Model file for the job. Use its own axes, mm. A direction names the side the tool comes from. Coordinates: 2 decimals unless noted, no trailing zeros. Write each loop counter-clockwise with the first axis right and the second up, starting at its lowest first coordinate (ties: lowest second). Pieces come first, ordered by that corner, then holes. Notation, with made-up numbers: (34.25, 33) - (52.25, 33) arc R17 cw to (52.25, 57) - close; hole circle Ø7 at (36.5, -26). An arc over 180 degrees is marked (long way). Put each result on its own line as item: value. Start each with the question number.
1. Saw through at B-B, the plane y = -3. Write the cut outline in (x, z).
2. Saw through at C-C, the plane y = -12. Write the cut outline in (x, z), plus the area to 3 significant figures.
3. Drop flat-ended pins along their axis: P1, Ø2, axis at x = -13.5, z = 2.5, coming from the +Y side; P2, Ø2.5, axis at x = -63, z = 1.5, coming from the +Y side; P3, Ø3.5, axis at y = -1, z = 1, coming from the +X side. Give the stop position or say it passes through.
4. Which spindle directions (+Z, -Z, +X, -X, +Y, -Y) get a long thin tool onto all of the face, cutting with end or side? Do faces 1 (the face through (-47.167, -18.974, 4.972)), 2 (the face through (-5, 16, 1)), 3 (the face through (-75, -20, 1)). Say none if no direction does.
5. Drill centre lines: L1, parallel to Y at x = -93.5, z = 0.75; L2, parallel to Y at x = -109, z = 1; L3, parallel to X at y = -22, z = 1. Where is each one in solid material? Low to high. Write a range as from..to.
6. Saw through at A-A, the plane x = -36.5. Write the cut outline in (y, z), plus the area to 3 significant figures.
7. Pull direction X, two halves, no side cores. Call faces 4 (the face through (-106.49, 16.92, 4.97)), 5 (the face through (-45.997, -15.181, 1.479)), 6 (the face through (-120, 16, 1)), 7 (the face through (5.416, 12.94, 1.479)): released by +X, released by -X, zero draft, split by the parting line, or undercut.
Autodesk Inventor part; units mm, degrees
ref_plane "YZ Plane" through (0, 0, 0) normal (1, 0, 0) x (0, 1, 0)
ref_plane "XZ Plane" through (0, 0, 0) normal (0, 1, 0) x (-1, 0, 0)
ref_plane "XY Plane" through (0, 0, 0) normal (0, 0, 1) x (1, 0, 0)
sketch "Sketch1" plane through (0, 0, 0) normal (0, 0, 1) x (1, 0, 0)
  circle A0 centre (1.5276, -12) radius 1.75
  circle A1 centre (1.5276, 0) radius 1.75
  circle A2 centre (1.5276, 12) radius 1.75
  arc A3 (1.5276, -16) -> (3.2181, -8.3748) centre (1.5276, -12) ccw
  line L0 (3.2181, -8.3748) -> (-2.4724, -5.7213)
  line L1 (1.5276, -16) -> (-60.6, -16)
  line L2 (11.3984, 0) -> (-64.1078, 0)
  line L3 (-60.6, 141.7) -> (-60.6, -41.7)
  line L4 (-2.4724, -5.7213) -> (-2.4724, 0)
  arc A4 (3.2181, 8.3748) -> (1.5276, 16) centre (1.5276, 12) ccw
  line L5 (3.2181, 8.3748) -> (-2.4724, 5.7213)
  line L6 (1.5276, 16) -> (-60.6, 16) construction
  line L7 (-2.4724, 5.7213) -> (-2.4724, 0)
  circle A5 centre (-32.0875, 25.9484) radius 1.6
  circle A6 centre (-44.5875, -20.9516) radius 1.6
  circle A7 centre (-109.5875, -20.9516) radius 1.6
  circle A8 centre (-109.5875, 17.8984) radius 1.6
  line L8 (-30.6, -16) -> (-40.6, -26)
  line L9 (-30.6, -16) -> (-16.4579, -16) construction
  line L10 (-40.6, -26) -> (-60.6, -26)
  line L11 (1.5276, 16) -> (-23.224, 16)
  line L12 (-23.224, 16) -> (-31.224, 24) construction
  line L13 (-23.224, 16) -> (-11.9103, 16) construction
  line L14 (-31.224, 24) -> (-109.7276, 24)
  line L15 (-109.7276, 24) -> (-117.7276, 16)
  circle A9 centre (-122.7276, -12) radius 1.75
  circle A10 centre (-122.7276, 0) radius 1.75
  circle A11 centre (-122.7276, 12) radius 1.75
  arc A12 (-124.4181, -8.3748) -> (-122.7276, -16) centre (-122.7276, -12) ccw
  arc A13 (-122.7276, 16) -> (-124.4181, 8.3748) centre (-122.7276, 12) ccw
  line L16 (-122.7276, 16) -> (-117.7276, 16)
  line L17 (-60.6, -26) -> (-112.7276, -26)
  line L18 (-112.7276, -26) -> (-122.7276, -16)
  line L19 (-124.4181, -8.3748) -> (-118.7276, -5.7213)
  line L20 (-118.7276, -5.7213) -> (-118.7276, 0)
  line L21 (-118.7276, 5.7213) -> (-118.7276, 0)
  line L22 (-124.4181, 8.3748) -> (-118.7276, 5.7213)
  line L23 (-11.9103, 16) -> (-25.5298, 29.6196)
  line L24 (-11.9103, 16) -> (7.3507, 16) construction
  line L25 (-25.5298, 29.6196) -> (-40.2322, 29.6196)
  line L26 (-40.2322, 29.6196) -> (-45.8517, 24)
  line L27 (-12.954, -10.4954) -> (-41.3116, -10.4954)
  line L28 (-41.3116, -10.4954) -> (-50.8162, -20)
  line L29 (-50.8162, -20) -> (-99.9221, -20)
  line L30 (-99.9221, -20) -> (-110.7276, -9.1945)
  line L31 (-110.7276, -9.1945) -> (-110.7276, 3.4171)
  line L32 (-110.7276, 3.4171) -> (-98.1447, 16)
  line L33 (-98.1447, 16) -> (-21.5239, 16)
  line L34 (-21.5239, 16) -> (-17.2785, 11.7546)
  line L35 (-17.2785, 11.7546) -> (-17.448, 11.7546)
  line L36 (-17.448, 11.7546) -> (-8.8369, 3.1435)
  line L37 (-8.8369, 3.1435) -> (-8.8369, -6.3783)
  line L38 (-8.8369, -6.3783) -> (-12.954, -10.4954)
  point P0 (0, 0)
extrude "Extrusion1" add sketch "Sketch1" along normal blind 3 contours L4 L0 A3 L1 L28 L27 L38 L37 L2 | L2 L37 L36 L35 L34 L11 A4 L5 L7 | L33 L32 L31 L30 L29 L3 L17 L18 A12 L19 L20 L21 L22 A13 L16 L15 L14 | L3 L14 L26 L25 L23 L11 L33 | L1 L8 L10 L3 L29 L28
sketch "Sketch2" plane through (0, 0, 3) normal (0, 0, 1) x (1, 0, 0)
  circle A0 centre (-32.0875, 25.9484) radius 1.6
  circle A1 centre (-44.5875, -20.9516) radius 1.6
  circle A2 centre (-109.5875, -20.9516) radius 1.6
  circle A3 centre (-109.5875, 17.8984) radius 1.6
  circle A4 centre (-109.5875, -20.9516) radius 3.25
  circle A5 centre (-109.5875, 17.8984) radius 3.25
  circle A6 centre (-32.0875, 25.9484) radius 3.25
  circle A7 centre (-44.5875, -20.9516) radius 1.6
  circle A8 centre (-44.5875, -20.9516) radius 3.25
  point P0 (0, 0)
  dimension "d15" = 6.5
  dimension "d16" = 6.5
  dimension "d17" = 6.5
  dimension "d18" = 6.5
extrude "Extrusion2" add sketch "Sketch2" along normal blind 4
properties part number "Motordriver_Adapter"
Final values:
1. outline: (-118.73, 0) - (-110.73, 0) - (-110.73, 3) - (-118.73, 3) - close; (-8.84, 0) - (-2.47, 0) - (-2.47, 3) - (-8.84, 3) - close
2. outline: (-126.73, 0) - (-124.48, 0) - (-124.48, 3) - (-126.73, 3) - close; (-120.98, 0) - (-107.92, 0) - (-107.92, 3) - (-120.98, 3) - close; (-42.82, 0) - (-0.22, 0) - (-0.22, 3) - (-42.82, 3) - close; (3.28, 0) - (5.53, 0) - (5.53, 3) - (3.28, 3) - close
2. area: 180 mm²
3. P1: stops at y = 18.59
3. P2: stops at y = 24
3. P3: stops at x = -2.47
4. face 1: +Z
4. face 2: +Z, -Z, +X, +Y
4. face 3: +Z, -Z
5. L1: y = -26..-20, 16..24
5. L2: y = -26..-22.44, -19.46..-10.92, 5.14..16.41, 19.39..24
5. L3: x = -116.73..-110.8, -108.38..-45.8, -43.38..-36.6
6. outline: (-21.9, 0) - (-10.5, 0) - (-10.5, 3) - (-21.9, 3) - close; (16, 0) - (29.62, 0) - (29.62, 3) - (16, 3) - close
6. area: 75.1 mm²
7. face 4: split by the parting line
7. face 5: undercut
7. face 6: zero draft
7. face 7: released by +X
